Autodesk Inventor part; units mm, degrees
ref_plane "YZ Plane" through (0, 0, 0) normal (1, 0, 0) x (0, 1, 0)
ref_plane "XZ Plane" through (0, 0, 0) normal (0, 1, 0) x (-1, 0, 0)
ref_plane "XY Plane" through (0, 0, 0) normal (0, 0, 1) x (1, 0, 0)
sketch "Sketch1" plane through (0, 0, 0) normal (0, 0, 1) x (1, 0, 0)
  arc A0 (9.5, -22.0397) -> (9.5, 22.0397) centre (0, 0) ccw
  line L0 (-9.5, 22) -> (-9.5, -22) construction
  line L1 (9.5, 22.0397) -> (9.5, -22.0397) construction
  line L2 (9.5, 22.0397) -> (9.5, 24)
  line L3 (9.5, 24) -> (-9.5, 24)
  line L4 (-9.5, 24) -> (-9.5, 22)
  line L5 (-9.5, 22) -> (-12.5, 22)
  line L6 (-12.5, 22) -> (-12.5, 28.5)
  arc A1 (17.5089, 23.75) -> (28.0178, 19) centre (28.0178, 33) ccw
  line L7 (28.0178, 19) -> (34.0178, 19)
  line L8 (34.0178, 19) -> (34.0178, -19)
  line L9 (9.5, -22.0397) -> (9.5, -24)
  line L10 (9.5, -24) -> (-9.5, -24)
  line L11 (-9.5, -24) -> (-9.5, -22)
  line L12 (-12.5, -22) -> (-12.5, -28.5)
  line L13 (-9.5, -22) -> (-12.5, -22)
  arc A2 (28.0178, -19) -> (17.5089, -23.75) centre (28.0178, -33) ccw
  line L14 (28.0178, -19) -> (34.0178, -19)
  line L15 (-12.5, 28.5) -> (7, 28.5)
  arc A3 (17.5089, 23.75) -> (7, 28.5) centre (7, 14.5) ccw
  line L16 (-12.5, -28.5) -> (7, -28.5)
  arc A4 (7, -28.5) -> (17.5089, -23.75) centre (7, -14.5) ccw
  point P0 (9.5, 0)
  point P1 (0, -24)
  point P2 (0, 24)
  point P3 (-2.75, 28.5)
  point P4 (-2.75, -28.5)
  dimension "d0" = 48
  dimension "d1" = 9.5
  dimension "d2" = 9.5
  dimension "d3" = 38
  dimension "d4" = 19
  dimension "d7" = 14
  dimension "d8" = 14
  dimension "d9" = 14
  dimension "d10" = 7
  dimension "d11" = 14
  dimension "d12" = 7
  dimension "d13" = 12.5
  dimension "d14" = 12.5
  dimension "d15" = 4.5
  dimension "d16" = 4.5
  dimension "d17" = 2
  dimension "d18" = 2
  dimension "d19" = 24
  dimension "d20" = 24
  dimension "d21" = 6
extrude "Extrusion1" add sketch "Sketch1" along normal mid plane 12
sketch "Sketch2" plane through (34.0178, -19, 6) normal (1, 0, 0) x (0, 0, -1)
  point P0 (6, 19)
  point P1 (6, 31.5)
  point P2 (6, 6.5)
  dimension "d31" = 25
  dimension "d32" = 12.5
hole "Hole1" at (34.0178, 12.5, 0) at (34.0178, -12.5, 0) direction (-1, 0, 0) diameter 4.134 end through all
sketch "Sketch3" plane through (-12.5, 28.5, 6) normal (0, 1, 0) x (1, 0, 0)
  line L0 (0, 12) -> (0, 0)
  point P0 (12.5, 6)
  point P1 (12.5, 6)
  point P2 (0, 6)
  point P3 (0, 6)
  dimension "d40" = 12.5
hole "Hole2" at (0, 28.5, 0) direction (0, -1, 0) diameter 6 depth 4.5
mirror "Mirror1" about plane through (0, 0, 0) normal (0, 1, 0) of "Hole2"
equation "\"d7\" = d5"
equation "\"d8\" = d5"
properties part number "102 new"
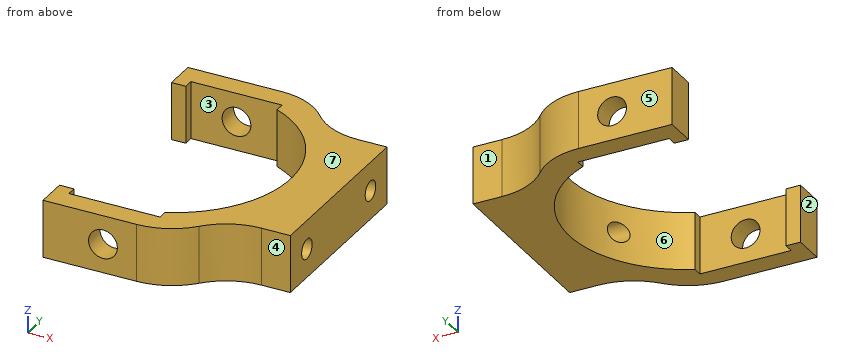
The model under review builds one solid part; all positions refer to its coordinate system, in mm. Face numbers are marked on the shaded views. A direction names the side the tool comes from. Round coordinates to 2 decimals unless told otherwise and drop trailing zeros. Loops run counter-clockwise (first coordinate to the right, second up) from the corner with the lowest first, then second, coordinate; pieces in that order, holes last. Notation, with made-up numbers: M 83,44 L 97,44 A24 ccw 97,82 Z; hole C 1.5,47 d3. An arc over 180 degrees is marked long. Answer as a JSON object with one key per item and string values.
(1) Draft analysis for pull direction Y (two halves, no side actions). For the marked faces 5, 6 and 7, state which applies: released by +Y, released by -Y, zero draft, split by the parting line, or undercut.
Resolved:
{"face 5": "released by +Y", "face 6": "undercut", "face 7": "zero draft"}
(2) Take a section at D-D on z = -1. Count the separate pieces of the cut face and the enclosed holes in it, and give its area (3 significant figures).
Resolved:
{"separate pieces": "5", "enclosed holes": "0", "area": "684 mm²"}
(3) Tool access review of the marked faces 1, 2, 3 and 4: name each direction out of +Z, -Z, +X, -X, +Y, -Y from which nothing blocks a thin tool from reaching the whole face with its end or side.
Resolved:
{"face 1": "+Z, -Z, +X, +Y", "face 2": "+Z, -Z, -X, +Y, -Y", "face 3": "+Z, -Z", "face 4": "+Z, -Z, +X, -Y"}
(4) Clearance check with flat-ended pins moving along their axes: P1, Ø6.5, axis at y = -12.5, z = 0, coming from the -X side; P2, Ø1, axis at y = 23.5, z = 0, coming from the +X side; P3, Ø0.6, axis at y = -23, z = 0, coming from the +X side; P4, Ø3.5, axis at x = 0, z = 0, coming from the +Y side. State where each tip first meets the part, or that it passes through.
Resolved:
{"P1": "x = 18.11", "P2": "x = 18.22", "P3": "x = 18.54", "P4": "through"}
(5) Take a section at A-A on x = -4.5. Give the boundary of the cut face in (y, z).
Resolved:
{"outline": "M -28.5,-6 L -24,-6 L -24,6 L -28.5,6 Z; M 24,-6 L 28.5,-6 L 28.5,6 L 24,6 Z"}
(6) To check wall thickness, follow line 1 along Y through (x, z) = (-6.5, -2.75); line 2 along Z through (x, y) = (0, 25.35); line 3 along Z through (x, y) = (23.5, 12.5). State the ranges of each line that lie inside material, in increasing order.
Resolved:
{"line 1": "-28.5 to -24, 24 to 28.5", "line 2": "-6 to -3, 3 to 6", "line 3": "-6 to -2.07, 2.07 to 6"}
(7) Take a section at B-B on y = 12.5. Give the boundary of the cut face in (x, z).
Resolved:
{"outline": "M 20.49,-6 L 34.02,-6 L 34.02,-2.07 L 20.49,-2.07 Z; M 20.49,2.07 L 34.02,2.07 L 34.02,6 L 20.49,6 Z"}
(8) Take a section at C-C on x = 29. Give the boundary of the cut face in (y, z).
Resolved:
{"outline": "M -19,-6 L 19,-6 L 19,6 L -19,6 Z; hole C -12.5,0 d4.13; hole C 12.5,0 d4.13"}
